Work out the finished part from the listing and answer in its coordinate system (mm). Give positions to 0.01 mm unless a question says otherwise; leave off trailing zeros. Loops run counter-clockwise (first coordinate to the right, second up) from the corner with the lowest first, then second, coordinate; pieces in that order, holes last. Notation, with made-up numbers: M 12,34.5 L 22,34.5 A22 cw 22,58.5 Z; hole C -24.5,-36.5 d5. An arc over 180 degrees is marked long. Answer in a Markdown table with one row per item. Add a question column.
from build123d import *

# Parameters (mm, degrees)
SKETCH_1_W          = 115.8
SKETCH_1_H          = 26.5
EXTRUDE_1_DEPTH     = 26.4
SKETCH_2_R          = 2
CUT_EXTRUDE_5_DEPTH = 106.070564596
SKETCH_3_W          = 26.5
SKETCH_3_H          = 26.4
CUT_EXTRUDE_6_DEPTH = 0.5
SKETCH_4_W          = 26.5
SKETCH_4_H          = 26.4
CUT_EXTRUDE_7_DEPTH = 0.5


with BuildPart() as part:
    # 草图1 → 凸台-拉伸1 (new body)
    with BuildSketch(Plane(origin=(0, 0, 0), x_dir=(1, 0, 0), z_dir=(0, 1, 0))):
        with Locations((42.656744125, -1.955418624)):
            Rectangle(SKETCH_1_W, SKETCH_1_H)
    extrude(amount=EXTRUDE_1_DEPTH)

    # 草图2 → 切除-拉伸5 (cut, through all)
    with BuildSketch(Plane(origin=(0, 26.4, 0), x_dir=(1, 0, 0), z_dir=(0, 1, 0))):
        with Locations(Location((-13.043255875, -1.955418624, 0), (0, 0, 270))):
            Circle(SKETCH_2_R)
        with Locations(Location((98.356744125, -1.955418624, 0), (0, 0, 270))):
            Circle(SKETCH_2_R)
    extrude(amount=-CUT_EXTRUDE_5_DEPTH, mode=Mode.SUBTRACT)

    # 草图3 → 切除-拉伸6 (cut)
    with BuildSketch(Plane(origin=(100.556744125, 0, 0), x_dir=(0, 0, -1), z_dir=(1, 0, 0))):
        with Locations((-1.955418624, 13.2)):
            Rectangle(SKETCH_3_W, SKETCH_3_H)
    extrude(amount=-CUT_EXTRUDE_6_DEPTH, mode=Mode.SUBTRACT)

    # 草图4 → 切除-拉伸7 (cut)
    with BuildSketch(Plane.ZY.offset(15.243255875)):
        with Locations((1.955418624, 13.2)):
            Rectangle(SKETCH_4_W, SKETCH_4_H)
    extrude(amount=-CUT_EXTRUDE_7_DEPTH, mode=Mode.SUBTRACT)


solid = part.part
(1) The mould has two halves that part along X. Classify faces 1 (the face through (42, 26.4, 2)), 2 (the face through (100.057, 13, 9)), 3 (the face through (-11.045, 13.385, 2.028)), 4 (the face through (96.36, 13.38, 1.88)): pulls with the +X half, pulls with the -X half, needs draft (parallel to the pull), parting line crosses it, or undercut.
(2) Section A-A, the plane z = 2 is taken. Determine the outline of the cut face in (x, y).
(3) Consider line 1 along X through (y, z) = (18.25, 1.5). Determine where the line is inside the solid, lowest interval first. Write a range as from..to.
Numbers:
| question | item | result |
|---|---|---|
| 1 | face 1 | needs draft |
| 1 | face 2 | pulls with the +X half |
| 1 | face 3 | undercut |
| 1 | face 4 | undercut |
| 2 | outline | M -11.04,0 L 96.36,0 L 96.36,26.4 L -11.04,26.4 Z |
| 3 | line 1 | x = -11.1..96.41 |
